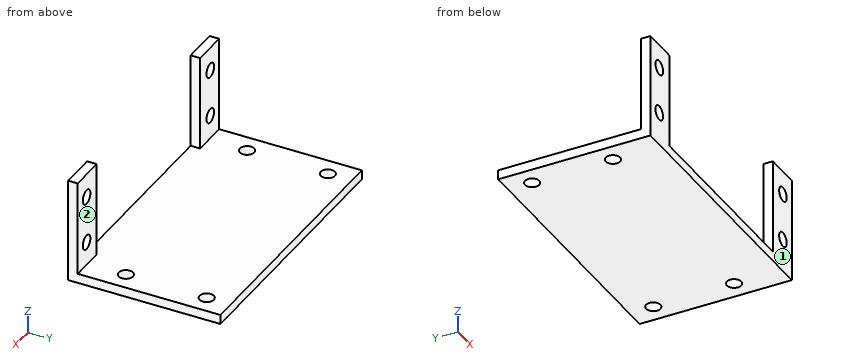
```python
from build123d import *

# Parameters (mm, degrees)
ESQUISSE1_W             = 56
ESQUISSE1_H             = 22
BOSS_EXTRU_1_DEPTH      = 2
ESQUISSE2_W             = 56
ESQUISSE2_H             = 2
BOSS_EXTRU_2_DEPTH      = 30
ESQUISSE3_W             = 41
ESQUISSE3_H             = 20
ENL_V_MAT_EXTRU_1_DEPTH = 20
ESQUISSE5_R             = 1.5
ENL_V_MAT_EXTRU_2_DEPTH = 20
ESQUISSE6_R             = 1.5
ENL_V_MAT_EXTRU_3_DEPTH = 20


with BuildPart() as part:
    # Esquisse1 → Boss.-Extru.1 (new body)
    with BuildSketch(Plane(origin=(0, 0, 0), x_dir=(1, 0, 0), z_dir=(0, 1, 0))):
        Rectangle(ESQUISSE1_W, ESQUISSE1_H)
    extrude(amount=BOSS_EXTRU_1_DEPTH)

    # Esquisse2 → Boss.-Extru.2 (add)
    with BuildSketch(Plane(origin=(0, 2, 0), x_dir=(1, 0, 0), z_dir=(0, 1, 0))):
        with Locations((0, 10)):
            Rectangle(ESQUISSE2_W, ESQUISSE2_H)
    extrude(amount=BOSS_EXTRU_2_DEPTH)

    # Esquisse3 → Enlèv. mat.-Extru.1 (cut)
    with BuildSketch(Plane(origin=(0, 2, 0), x_dir=(1, 0, 0), z_dir=(0, 1, 0))):
        with Locations((0, -1)):
            Rectangle(ESQUISSE3_W, ESQUISSE3_H)
    extrude(amount=-ENL_V_MAT_EXTRU_1_DEPTH, mode=Mode.SUBTRACT)

    # Esquisse5 → Enlèv. mat.-Extru.2 (cut)
    with BuildSketch(Plane(origin=(0, 2, 0), x_dir=(1, 0, 0), z_dir=(0, 1, 0))):
        with Locations((-24.5, 4)):
            Circle(ESQUISSE5_R)
        with Locations((-24.5, -6)):
            Circle(ESQUISSE5_R)
        with Locations((24.5, 4)):
            Circle(ESQUISSE5_R)
        with Locations((24.5, -6)):
            Circle(ESQUISSE5_R)
    extrude(amount=-ENL_V_MAT_EXTRU_2_DEPTH, mode=Mode.SUBTRACT)

    # Esquisse6 → Enlèv. mat.-Extru.3 (cut)
    with BuildSketch(Plane(origin=(0, 0, -11), x_dir=(-1, 0, 0), z_dir=(0, 0, -1))):
        with Locations((-24, 27)):
            Circle(ESQUISSE6_R)
        with Locations((-24, 10)):
            Circle(ESQUISSE6_R)
        with Locations((24, 10)):
            Circle(ESQUISSE6_R)
        with Locations((24, 27)):
            Circle(ESQUISSE6_R)
    extrude(amount=-ENL_V_MAT_EXTRU_3_DEPTH, mode=Mode.SUBTRACT)


solid = part.part
```
Geometry: final body of the model. Coordinates: model frame, mm. Face numbers are marked on the shaded views. A direction names the side the tool comes from. Round coordinates to 2 decimals unless told otherwise and drop trailing zeros. Write each loop counter-clockwise with the first axis right and the second up, starting at its lowest first coordinate (ties: lowest second). Pieces come first, ordered by that corner, then holes. Notation, with made-up numbers: M 33.5,-37 L 78.5,-37 A23 ccw 78.5,-10 Z; hole C 14.25,46.25 d8. An arc over 180 degrees is marked long. Answer in a Markdown table with one row per item. Add a question column.
(1) Contact query for flat-ended pins moving along their axis: pin 1 (4 mm diameter, centred on x = -24, y = 27, fed in from +Z); pin 2 (3 mm diameter, centred on x = 21.5, z = 3.5, fed in from -Y); pin 3 (8 mm diameter, centred on x = -23.5, z = -2, fed in from +Y). Output: stop coordinate, or through.
(2) Ray query, L1, parallel to Z at x = 24.5, y = 1.3; L2, parallel to Y at x = 24, z = -10.1; L3, parallel to Z at x = -7, y = 25. Return the intervals inside material, ascending.
(3) Cut plane B-B, the plane y = 27. Return the cut outline in (x, z).
(4) Cut plane D-D, the plane x = -24. Return the cut outline in (y, z), then the cut area to 3 significant figures.
(5) Reachability of the marked faces 1 and 2 from +Z, -Z, +X, -X, +Y, -Y: full face, straight path, thin tool, end or side. Return the list, or none.
(6) Cut plane A-A, the plane z = 3. Return the cut outline in (x, y).
(7) Cut plane C-C, the plane z = 6. Return the cut outline in (x, y).
Established:
| question | item | result |
|---|---|---|
| 1 | pin 1 | z = -9 |
| 1 | pin 2 | y = 0 |
| 1 | pin 3 | y = 2 |
| 2 | L1 | -11 to -5.5, -2.5 to 4.5, 7.5 to 11 |
| 2 | L2 | 0 to 8.5, 11.5 to 25.5, 28.5 to 32 |
| 2 | L3 | -11 to -9 |
| 3 | outline | M -28,-11 L -25.5,-11 L -25.5,-9 L -28,-9 Z; M -22.5,-11 L 22.5,-11 L 22.5,-9 L -22.5,-9 Z; M 25.5,-11 L 28,-11 L 28,-9 L 25.5,-9 Z |
| 4 | outline | M 0,-11 L 8.5,-11 L 8.5,-9 L 2,-9 L 2,-5.41 L 0,-5.41 Z; M 0,-2.59 L 2,-2.59 L 2,4.59 L 0,4.59 Z; M 0,7.41 L 2,7.41 L 2,11 L 0,11 Z; M 11.5,-11 L 25.5,-11 L 25.5,-9 L 11.5,-9 Z; M 28.5,-11 L 32,-11 L 32,-9 L 28.5,-9 Z |
| 4 | area | 80.7 mm² |
| 5 | face 1 | +Z, -Z, +X, -X, -Y |
| 5 | face 2 | +Z, +X, -X, +Y |
| 6 | outline | M -28,0 L -20.5,0 L -20.5,2 L -28,2 Z; M 20.5,0 L 28,0 L 28,2 L 20.5,2 Z |
| 7 | outline | M -28,0 L -26,0 L -26,2 L -28,2 Z; M -23,0 L -20.5,0 L -20.5,2 L -23,2 Z; M 20.5,0 L 23,0 L 23,2 L 20.5,2 Z; M 26,0 L 28,0 L 28,2 L 26,2 Z |
